For this review, use the dimensioned drawing (mm, ordinates from the lowest corner) and the shaded views. Coordinates: 2 decimals unless noted, no trailing zeros. Order: outer loops, then holes, each group sorted by start corner. A loop starts at its lowest first (then second) coordinate and runs counter-clockwise, first axis right, second up. Notation, with made-up numbers: M -0.75,-20 L 55.25,-20 A27 cw 55.25,9 Z; hole C 7,50.5 d1. An arc over 180 degrees is marked long. Answer in a Markdown table with one row per item.
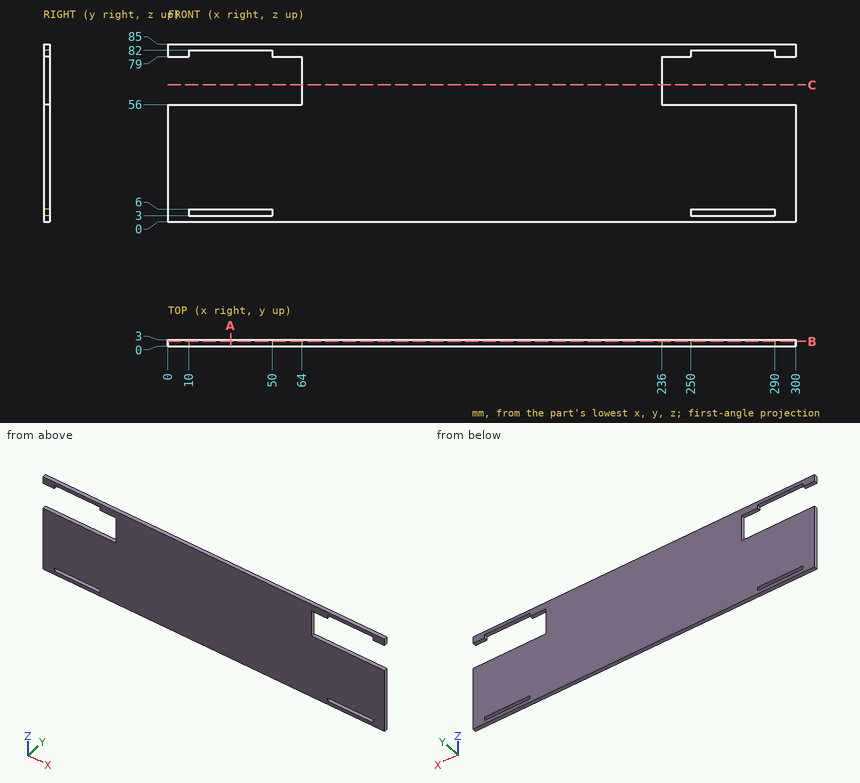
(1) Add section C-C, the plane z = 65.5. Give the boundary of the cut face in (x, y).
Return value:
| item | result |
|---|---|
| outline | M 64,0 L 236,0 L 236,3 L 64,3 Z |
(2) For line 1 along Z through (x, y) = (278, 2.85); line 2 along X through (y, z) = (1.85, 79.5); line 3 along X through (y, z) = (0.5, 74), list the stretches that pass through material, from the lowest coordinate up. Write a range as from..to.
Return value:
| item | result |
|---|---|
| line 1 | z = 0..3, 6..56, 82..85 |
| line 2 | x = 0..10, 50..250, 290..300 |
| line 3 | x = 64..236 |
(3) Add section A-A, the plane x = 30. Give the boundary of the cut face in (y, z).
Return value:
| item | result |
|---|---|
| outline | M 0,0 L 3,0 L 3,3 L 0,3 Z; M 0,6 L 3,6 L 3,56 L 0,56 Z; M 0,82 L 3,82 L 3,85 L 0,85 Z |
(4) Add section B-B, the plane y = 2.3. Give the boundary of the cut face in (x, z).
Return value:
| item | result |
|---|---|
| outline | M 0,0 L 300,0 L 300,56 L 236,56 L 236,79 L 250,79 L 250,82 L 290,82 L 290,79 L 300,79 L 300,85 L 0,85 L 0,79 L 10,79 L 10,82 L 50,82 L 50,79 L 64,79 L 64,56 L 0,56 Z; hole M 10,3 L 50,3 L 50,6 L 10,6 Z; hole M 250,3 L 290,3 L 290,6 L 250,6 Z |
(5) Insertion check: pin 1 Ø1.5 at (x, y) = (26, 2) entering from -Z; pin 2 Ø0.9 at (y, z) = (1, 66) entering from -X. Each pin has a flat end and moves straight along its axis. Give the tip position at first contact, or say it passes through.
Return value:
| item | result |
|---|---|
| pin 1 | stops at z = 0 |
| pin 2 | stops at x = 64 |
